Could you check a few things on this model? Use its own coordinates, in mm. A direction names the side the tool comes from. Round coordinates to 2 decimals unless told otherwise and drop trailing zeros. Order: outer loops, then holes, each group sorted by start corner. A loop starts at its lowest first (then second) coordinate and runs counter-clockwise, first axis right, second up. Notation, with made-up numbers: (67.25, -32.75) - (113.25, -32.75) arc R35 ccw to (113.25, 3.25) - close; hole circle Ø5 at (-28, 21). An arc over 180 degrees is marked (long way). Return JSON: item names as keys, results as strings. Group by question number.
Autodesk Inventor part; units mm, degrees
ref_plane "Start plane" through (0, 0, -17.5) normal (0, 0, 1) x (1, 0, 0)
ref_plane "End plane" through (0, 0, 817.5) normal (0, 0, 1) x (1, 0, 0)
ref_plane "Work Plane7" through (10, 0, -17.5) normal (0, 0, -1) x (-1, 0, 0)
ref_plane "Start plane" through (0, 0, -17.5) normal (0, 0, 1) x (1, 0, 0)
ref_plane "End plane" through (0, 0, 817.5) normal (0, 0, 1) x (1, 0, 0)
sketch "Sketch" plane through (0, 0, 0) normal (0, 0, 1) x (1, 0, 0)
  line L0 (-17.5, -14.3) -> (-17.5, 14.3)
  line L1 (-14.3, 17.5) -> (14.3, 17.5)
  line L2 (17.5, 14.3) -> (17.5, -14.3)
  line L3 (14.3, -17.5) -> (-14.3, -17.5)
  arc A0 (-17.5, -14.3) -> (-14.3, -17.5) centre (-14.3, -14.3) ccw
  arc A1 (-14.3, 17.5) -> (-17.5, 14.3) centre (-14.3, 14.3) ccw
  arc A2 (17.5, 14.3) -> (14.3, 17.5) centre (14.3, 14.3) ccw
  arc A3 (14.3, -17.5) -> (17.5, -14.3) centre (14.3, -14.3) ccw
  arc A4 (-14.3, 15.9) -> (-15.9, 14.3) centre (-14.3, 14.3) ccw
  line L4 (-14.3, 15.9) -> (14.3, 15.9)
  arc A5 (15.9, 14.3) -> (14.3, 15.9) centre (14.3, 14.3) ccw
  line L5 (15.9, 14.3) -> (15.9, -14.3)
  arc A6 (14.3, -15.9) -> (15.9, -14.3) centre (14.3, -14.3) ccw
  line L6 (14.3, -15.9) -> (-14.3, -15.9)
  arc A7 (-15.9, -14.3) -> (-14.3, -15.9) centre (-14.3, -14.3) ccw
  line L7 (-15.9, -14.3) -> (-15.9, 14.3)
  line L8 (0, 25.4278) -> (0, -25.4278) construction
  line L9 (-25.4278, 0) -> (25.4278, 0) construction
  dimension "d7" = 3.2
  dimension "d10" = 35
  dimension "d11" = 35
  dimension "d12" = 1.6
  dimension "d15" = 17.5
  dimension "d16" = 17.5
extrude "Body" add sketch "Sketch" along normal up to surface (835 mm away) from surface at -17.5
sketch "Sketch3" plane through (0, 0, 0) normal (0, 0, 1) x (1, 0, 0)
  line L0 (0, 0) -> (10, 0)
ref_plane "Work Plane3" through (0, 0, 0) normal (0, -1, 0) x (1, 0, 0)
sketch "Sketch4" plane through (0, 0, 0) normal (0, -1, 0) x (1, 0, 0)
  line L0 (-2, -17.5) -> (12, -17.5)
  line L1 (-2, 817.5) -> (12, 817.5)
  dimension "d18" = 835
ref_plane "Work Plane7" through (10, 0, -17.5) normal (0, 0, -1) x (-1, 0, 0)
split "Split4" plane through (10, 0, -17.5) removes the side toward (0, 0, -1)
ref_plane "Work Plane8" through (0, -17.5, -17.5) normal (0, 0.7071, -0.7071) x (1, 0, 0)
split "Split5" plane through (0, -17.5, -17.5) removes the side toward (0, 0.7071, -0.7071)
ref_plane "Work Plane9" through (0, -17.5, 817.5) normal (0, 0.7071, 0.7071) x (1, 0, 0)
split "Split6" plane through (0, -17.5, 817.5) removes the side toward (0, 0.7071, 0.7071)
sketch "Sketch5" plane through (17.5, -14.3, 814.3) normal (1, 0, 0) x (0, 0, -1)
  line L0 (28.6, 28.6) -> (0, 0) construction
  line L1 (0, 0) -> (828.6, 0) construction
  line L2 (828.6, 0) -> (800, 28.6) construction
  line L3 (28.6, 28.6) -> (200, 28.6) construction
  line L4 (721.8, 0) -> (721.8, 28.6) construction
  line L5 (28.6, 28.6) -> (800, 28.6) construction
  line L6 (796.8, 496.8) -> (796.8, 31.8) construction
  line L7 (721.8, 14.3) -> (610.3, 14.3) construction
  line L8 (610.3, 28.6) -> (610.3, 0) construction
  line L9 (31.8, 96.8) -> (31.8, 31.8) construction
  line L10 (106.8, 28.6) -> (106.8, 0) construction
  line L11 (106.8, 14.3) -> (218.3, 14.3) construction
  line L12 (218.3, 28.6) -> (218.3, 0) construction
  line L13 (200, 28.6) -> (200, 14.3)
  line L14 (228.6, 28.6) -> (400, 28.6)
  line L15 (228.6, 28.6) -> (228.6, 14.3)
  line L16 (228.6, 14.3) -> (200, 14.3)
  line L17 (400, 28.6) -> (400, 14.3)
  line L18 (428.6, 28.6) -> (600, 28.6)
  line L19 (428.6, 28.6) -> (428.6, 14.3)
  line L20 (428.6, 14.3) -> (400, 14.3)
  line L21 (600, 28.6) -> (600, 14.3)
  line L22 (628.6, 28.6) -> (800, 28.6)
  line L23 (628.6, 28.6) -> (628.6, 14.3)
  line L24 (628.6, 14.3) -> (600, 14.3)
  point P0 (814.3, 14.3)
  dimension "d19" = 75
  dimension "d20" = 111.5
  dimension "d22" = 75
  dimension "d23" = 111.5
hole "Hole1" at (17.5, 0, 92.5) at (17.5, 0, 204) at (17.5, 0, 596) at (17.5, 0, 707.5) direction (-1, 0, 0) diameter 10 end through all
equation "\"d7\" = G_IR"
equation "\"d10\" = G_H"
equation "\"d11\" = G_W"
equation "\"d12\" = G_T"
equation "\"d15\" = 0.5 * d10"
equation "\"d16\" = 0.5 * d11"
equation "\"d3\" = G_L"
equation "\"G_W\" = 35"
equation "\"G_H\" = 35"
equation "\"G_T\" = 1.6"
equation "\"G_IR\" = 3.2"
equation "\"G_L\" = d18"
equation "\"G_OFFSET_START\" = 17.5"
equation "\"G_OFFSET_END\" = 17.5"
equation "\"d13\" = -G_OFFSET_START"
equation "\"d14\" = G_OFFSET_END + B_L"
properties part number "AS 1163 - C350L0 35x35x1.6 SHS - 835" material "Steel, Mild"
1) Will these pins go through, and if not, where does the flat tip stop? pin 1 (11.5 mm diameter, centred on y = 0, z = 204, fed in from +X); pin 2 (8 mm diameter, centred on y = 0, z = 92.5, fed in from +X).
2) We'd pull the mould along Y, two halves only. Please class faces 1 (the flat face through (-17.5, 0, 394)), 2 (the flat face through (17, -1, 801)), 3 (the flat face through (0, -15.9, 394)), 4 (the flat face through (15.9, 0, 394)): +Y half, -Y half, draft (parallel to the pull), parting line (faces both ways), or undercut.
3) If I drill on line 1 along Y through (x, z) = (-7.5, 442.5); line 2 along Y through (x, z) = (-15, 214.5), over which ranges is the centre line in solid material (lowest first)? Write a range as from..to.
4) For faces 5 (the flat face through (0, -17.5, 394)), 6 (the flat face through (0, 15.9, 395)), which set-ups out of +Z, -Z, +X, -X, +Y, -Y let a thin tool reach every point of the face, with its end or its side?
5) I want a section at B-B, the plane z = 556. List the corners of the cut face in (x, y) for me, plus the area to 3 significant figures.
6) I want a section at A-A, the plane x = 5.5. List the corners of the cut face in (y, z) for me.
Outcome:
{
 "1": {"pin 1": "x = 17.5", "pin 2": "through"},
 "2": {"face 1": "draft", "face 2": "+Y half", "face 3": "undercut", "face 4": "undercut"},
 "3": {"line 1": "-17.5..-15.9, 15.9..17.5", "line 2": "-17.42..-15.74, 15.74..17.42"},
 "4": {"face 5": "+Z, -Z, +X, -X, -Y", "face 6": "+Z, -Z"},
 "5": {"outline": "(-17.5, -14.3) arc R3.2 ccw to (-14.3, -17.5) - (14.3, -17.5) arc R3.2 ccw to (17.5, -14.3) - (17.5, 14.3) arc R3.2 ccw to (14.3, 17.5) - (-14.3, 17.5) arc R3.2 ccw to (-17.5, 14.3) - close; hole (-15.9, -14.3) arc R1.6 ccw to (-14.3, -15.9) - (14.3, -15.9) arc R1.6 ccw to (15.9, -14.3) - (15.9, 14.3) arc R1.6 ccw to (14.3, 15.9) - (-14.3, 15.9) arc R1.6 ccw to (-15.9, 14.3) - close", "area": "207 mm^2"},
 "6": {"outline": "(-17.5, -17.5) - (-15.9, -15.9) - (-15.9, 815.9) - (-17.5, 817.5) - close; (15.9, 15.9) - (17.5, 17.5) - (17.5, 782.5) - (15.9, 784.1) - close"}
}
